The listing builds one solid part. Answer for the finished solid, in the listing's coordinates (mm). A direction names the side the tool comes from. Coordinates: 2 decimals unless noted, no trailing zeros. Write each loop counter-clockwise with the first axis right and the second up, starting at its lowest first coordinate (ties: lowest second). Pieces come first, ordered by that corner, then holes.
from build123d import *

# Parameters (mm, degrees)
F0_R     = 14.7481793899
F1_DEPTH = 3
F1_TAPER = -3
F2_W     = 2.8173960745
F2_H     = 3.8187131286
F2_W_2   = 2.8887987137
F3_DEPTH = 7
F4_W     = 5.9206429869
F4_H     = 3.8187131286
F4_W_2   = 5.9958791826
F4_H_2   = 3.9352546446
F5_DEPTH = 2
F6_W     = 3.1207427382
F6_H     = 3.8840055931
F7_DEPTH = 7
F8_W     = 3.1032469124
F8_H     = 3.8187131286
F9_DEPTH = 7


with BuildPart() as f1:
    # F0 (on Top) → F1 (new body)
    with BuildSketch(Plane.XY):
        Circle(F0_R)
    extrude(amount=F1_DEPTH, taper=F1_TAPER)

    # F2 (on face) → F3 (join)
    with BuildSketch(Plane.XY.offset(3)):
        with Locations((-4.1453484446, 0)):
            Rectangle(F2_W, F2_H)
        with Locations((3.9267931134, 0)):
            Rectangle(F2_W_2, F2_H)
    extrude(amount=F3_DEPTH)

    # F4 (on face) → F5 (join)
    with BuildSketch(Plane.XY.offset(10)):
        with Locations((-5.6969719008, 0)):
            Rectangle(F4_W, F4_H)
        with Locations((5.4939956171, -0.0070217066)):
            Rectangle(F4_W_2, F4_H_2)
    extrude(amount=F5_DEPTH)

    # F6 (on face) → F7 (join)
    with BuildSketch(Plane(origin=(0, 0, 10), x_dir=(1, 0, 0), z_dir=(0, 0, -1))):
        with Locations((6.9315638393, 0.0326462323)):
            Rectangle(F6_W, F6_H)
    extrude(amount=F7_DEPTH)

    # F8 (on face) → F9 (join)
    with BuildSketch(Plane(origin=(0, 0, 10), x_dir=(1, 0, 0), z_dir=(0, 0, -1))):
        with Locations((-7.105669938, 0)):
            Rectangle(F8_W, F8_H)
    extrude(amount=F9_DEPTH)


solid = f1.part
Q1. Find the intervals of material crossed by probe 1 along Y at (x, z) = (-7.5, 10); probe 2 along Z at (x, y) = (-6, 9.5); probe 3 along X at (y, z) = (0.5, 11.25), in increasing order.
Answers below:
probe 1: y = -1.91 to 1.91
probe 2: z = 0 to 3
probe 3: x = -8.66 to -2.74, 2.5 to 8.49
Q2. The part is cut by section A-A, the plane z = 5.25. Write down the section's boundary in (x, y), then the cut area to 3 significant figures.
Answers below:
outline: (-8.66, -1.91) - (-2.74, -1.91) - (-2.74, 1.91) - (-8.66, 1.91) - close; (2.48, -1.91) - (5.37, -1.91) - (5.37, -1.97) - (8.49, -1.97) - (8.49, 1.91) - (2.48, 1.91) - close
area: 45.8 mm2
Q3. Determine the mould class of faces 1 (the face through (5, 0, 12)), 2 (the face through (14.11, 4.44, 0.85)), 3 (the face through (4, -1.909, 6)) for opening direction Z: released by +Z, released by -Z, zero draft, split by the parting line, or undercut.
Answers below:
face 1: released by +Z
face 2: released by -Z
face 3: undercut
Q4. The part is cut by section B-B, the plane x = 0. Write down the section's boundary in (y, z).
Answers below:
outline: (-14.91, 3) - (-14.75, 0) - (14.75, 0) - (14.91, 3) - close
Q5. Which of the six approach directions +Z, -Z, +X, -X, +Y, -Y give full straight-line access (tool end or side, diameter ignored) to faces 4 (the face through (-2.737, 0, 7)), 5 (the face through (6, -1.975, 9)), 6 (the face through (-6, -1.909, 8))?
Answers below:
face 4: +Z, +Y, -Y
face 5: +Z, +X, -X, -Y
face 6: +Z, -X, -Y
Q6. Given pin 1 (1 mm diameter, centred on x = -5.5, z = 9, fed in from +Y); pin 2 (1.1 mm diameter, centred on y = 0, z = 6, fed in from -X); pin 3 (0.9 mm diameter, centred on x = 4.5, z = 5, fed in from -Y); pin 4 (1.5 mm diameter, centred on y = -6.5, z = 5, fed in from +X), each flat-ended and moving along its own axis, determine where each tip first touches the part or whether it passes through.
Answers below:
pin 1: stops at y = 1.91
pin 2: stops at x = -8.66
pin 3: stops at y = -1.91
pin 4: passes through
